from build123d import *

# Parameters (mm, degrees)
SKETCH_2_W          = 2
SKETCH_2_H          = 2.409546764
CUT_EXTRUDE_1_DEPTH = 5


with BuildPart() as part:
    # 草圖1 → 旋轉1 (revolve)
    with BuildSketch(Plane.XY, mode=Mode.PRIVATE) as revolve_1_sk:
        with BuildLine():
            Line((-4, 12.5), (-4, 2.5))
            Line((-4, 2.5), (-1.834936491, 1.25))
            Line((-1.834936491, 1.25), (0, 1.25))
            Line((0, 1.25), (0, 13.5))
            ThreePointArc((0, 13.5), (-2.061552813, 13.246211251), (-4, 12.5))
        make_face()
    revolve(revolve_1_sk.sketch.rotate(Axis((0, 0, 0), (0, 1, 0)), 270), axis=Axis((0, 0, 0), (0, 1, 0)))

    # 草圖2 → 除料-伸長1 (cut, symmetric)
    with BuildSketch(Plane.XY):
        with Locations((0, 12.704773382)):
            Rectangle(SKETCH_2_W, SKETCH_2_H)
    extrude(amount=CUT_EXTRUDE_1_DEPTH, both=True, mode=Mode.SUBTRACT)


solid = part.part
Source: CAD feature listing. Evaluate the final solid. Frame: model axes, mm. Give positions to 0.01 mm unless a question says otherwise; leave off trailing zeros. Write each loop counter-clockwise with the first axis right and the second up, starting at its lowest first coordinate (ties: lowest second). Pieces come first, ordered by that corner, then holes. Notation, with made-up numbers: M 43,-22 L 60,-22 A28 ccw 60,9 Z; hole C 42.25,8.5 d9. An arc over 180 degrees is marked long. Answer as a JSON object with one key per item and string values.
Q1. Ray query, line 1 along Y through (x, z) = (0, -1.5); line 2 along Z through (x, y) = (-1, 2.75); line 3 along X through (y, z) = (12, -2.25). Return the intervals inside material, ascending.
Geometry check:
{"line 1": "y = 1.25 to 11.5", "line 2": "z = -3.87 to 3.87", "line 3": "x = -3.31 to -1, 1 to 3.31"}
Q2. Mould query, pull axis X, two halves, no side actions, for faces 1 (the face through (0, 1.25, 0)), 2 (the face through (1, 12, 0)), 3 (the face through (1.532, 7.43, -3.695)). Classes: +X half, -X half, draft (parallel to the pull), parting line (faces both ways), or undercut.
Geometry check:
{"face 1": "draft", "face 2": "undercut", "face 3": "parting line"}
Q3. Contact query for flat-ended pins moving along their axis: P1, Ø1.6, axis at x = -0.5, z = -1, coming from the +Y side; P2, Ø1, axis at y = 7.5, z = -2, coming from the -X side; P3, Ø1, axis at x = -2, z = 1.5, coming from the -Y side. Output: stop coordinate, or through.
Geometry check:
{"P1": "stops at y = 13.43", "P2": "stops at x = -3.71", "P3": "stops at y = 1.35"}
Q4. Cut plane C-C, the plane y = 4.5. Return the cut outline in (x, z).
Geometry check:
{"outline": "C 0,0 d8"}
Q5. Cut plane B-B, the plane x = 0. Return the cut outline in (y, z).
Geometry check:
{"outline": "M 1.25,-1.83 L 2.5,-4 L 11.5,-4 L 11.5,4 L 2.5,4 L 1.25,1.83 Z"}
Q6. Cut plane A-A, the plane z = 0. Return the cut outline in (x, y), then the cut area to 3 significant figures.
Geometry check:
{"outline": "M -4,2.5 L -1.83,1.25 L 1.83,1.25 L 4,2.5 L 4,12.5 A8.5 ccw 1,13.44 L 1,11.5 L -1,11.5 L -1,13.44 A8.5 ccw -4,12.5 Z", "area": "88.7 mm^2"}
